Design review of the part built by this model. Coordinates are the model's own, in mm. A direction names the side the tool comes from. Coordinates: 2 decimals unless noted, no trailing zeros.
Q1. The part is to be moulded in two halves that separate along X. For faces 4 (the cylindrical face through (8.672, 11.794, 5.267)), 5 (the flat face through (-13, 0, 5)), 6 (the flat face through (-5, 0, 13)), say which applies: released by +X, released by -X, zero draft, split by the parting line, or undercut.
Q2. For faces 1 (the flat face through (-5, 15, 12)), 2 (the cylindrical face through (-5.351, -21.323, 5.429)), 3 (the flat face through (9.4, 1.4, 10)), list the 3-axis set-ups (+Z, -Z, +X, -X, +Y, -Y) from which the entire face can be reached by the end or side of a thin tool; tool diameter is ignored.
Q3. For L1, parallel to X at y = 2, z = 6.75; L2, parallel to Z at x = -10.75, y = -18.5; L3, parallel to Y at x = -5, z = 6.25, list the stretches that pass through material, from the lowest coordinate up.
Q4. For pin 1 Ø3 at (x, y) = (-5, 24) entering from +Z; pin 2 Ø1.3 at (y, z) = (4, 11.5) entering from -X; pin 3 Ø1.5 at (x, z) = (8, 6.5) entering from +Y; pin 4 Ø2 at (x, z) = (7, 6.5) entering from +Y, all flat-tipped, find the tip position at first contact; note any pin that passes through.
Q5. Take a section at A-A, the plane x = -5. State how many separate pieces and enclosed holes the cut face has, plus the area to 3 significant figures.
from build123d import *

# Parameters (mm, degrees)
SKETCH1_R           = 2.7
BOSS_EXTRUDE1_DEPTH = 11
SKETCH2_W           = 6.5
SKETCH2_H           = 30
BOSS_EXTRUDE2_DEPTH = 2
SKETCH3_W           = 7.8
SKETCH3_H           = 35.5
BOSS_EXTRUDE3_DEPTH = 1
FILLET1_R           = 5
FILLET2_R           = 0.45
FILLET3_R           = 0.8
FILLET4_R           = 0.65
FILLET5_R           = 1.85
CHAMFER1_SIZE       = 0.4


with BuildPart() as part:
    # Sketch1 → Boss-Extrude1 (new body)
    with BuildSketch(Plane.XY):
        Polygon((-13, -30), (-13, 30), (13, 28.375), (13, -28.375), align=None)
        with Locations((-5, -24)):
            Circle(SKETCH1_R, mode=Mode.SUBTRACT)
        with Locations((-5, 24)):
            Circle(SKETCH1_R, mode=Mode.SUBTRACT)
        Polygon((3.2, -17.75), (3.2, -12.35), (9.2, -12.35), (9.2, 12.35), (3.2, 12.35), (3.2, 17.75), (4.5, 17.75), (4.5, 15.547994765), (5.34, 14.15), (8.29, 14.15), (9.79, 15.65), (11, 15.65), (11, -15.65), (9.79, -15.65), (8.29, -14.15), (5.34, -14.15), (4.5, -15.547994765), (4.5, -17.75), align=None, mode=Mode.SUBTRACT)
    extrude(amount=BOSS_EXTRUDE1_DEPTH)

    # Sketch2 → Boss-Extrude2 (add)
    with BuildSketch(Plane.XY.offset(11)):
        with Locations((-5, 0)):
            Rectangle(SKETCH2_W, SKETCH2_H)
    extrude(amount=BOSS_EXTRUDE2_DEPTH)

    # Sketch3 → Boss-Extrude3 (add)
    with BuildSketch(Plane.XY.offset(11)):
        with Locations((7.1, 0)):
            Rectangle(SKETCH3_W, SKETCH3_H)
    extrude(amount=-BOSS_EXTRUDE3_DEPTH)

    # Fillet1
    fillet1_edges = [part.edges().sort_by_distance(p)[0] for p in [
        (-13, -30, 5.5),
        (-13, 30, 5.5),
        (13, 28.375, 5.5),
        (13, -28.375, 5.5),
    ]]
    fillet(fillet1_edges, radius=FILLET1_R)

    # Fillet2
    fillet2_edges = [part.edges().sort_by_distance(p)[0] for p in [
        (3.2, 17.75, 5),
        (4.5, 17.75, 5),
        (4.5, -17.75, 5),
        (3.2, -17.75, 5),
    ]]
    fillet(fillet2_edges, radius=FILLET2_R)

    # Fillet3
    fillet3_edges = [part.edges().sort_by_distance(p)[0] for p in [
        (5.34, 14.15, 5),
        (5.34, -14.15, 5),
        (-8.25, 15, 12),
        (-8.25, -15, 12),
        (-1.75, -15, 12),
        (-1.75, 15, 12),
    ]]
    fillet(fillet3_edges, radius=FILLET3_R)

    # Fillet4
    fillet4_edges = [part.edges().sort_by_distance(p)[0] for p in [
        (3.2, 12.35, 5),
        (3.2, -12.35, 5),
    ]]
    fillet(fillet4_edges, radius=FILLET4_R)

    # Fillet5
    fillet5_edges = [part.edges().sort_by_distance(p)[0] for p in [
        (9.2, -12.35, 5),
        (9.2, 12.35, 5),
    ]]
    fillet(fillet5_edges, radius=FILLET5_R)

    # Chamfer1
    chamfer1_edges = [part.edges().sort_by_distance(p)[0] for p in [
        (-7.7, -24, 0),
        (-7.7, -24, 11),
        (0.311891431, -29.168006786, 0),
        (0.311891431, -29.168006786, 11),
        (-13, 0, 0),
        (0.311891431, 29.168006786, 0),
        (13, 0, 0),
        (-11.423488195, 28.321880084, 0),
        (11.644136191, 27.101232088, 0),
        (11.644136191, -27.101232088, 0),
        (-11.423488195, -28.321880084, 0),
        (-13, 0, 11),
        (13, 0, 11),
        (0.311891431, 29.168006786, 11),
        (-11.423488195, 28.321880084, 11),
        (-7.7, 24, 0),
        (11.644136191, 27.101232088, 11),
        (11.644136191, -27.101232088, 11),
        (-11.423488195, -28.321880084, 11),
        (-7.7, 24, 11),
        (3.85, 17.75, 0),
        (3.2, 15.15, 0),
        (3.85, -17.75, 0),
        (4.5, -16.423997383, 0),
        (4.368198052, 17.618198052, 0),
        (3.331801948, 17.618198052, 0),
        (4.368198052, -17.618198052, 0),
        (3.331801948, -17.618198052, 0),
        (-5, -15, 13),
        (-8.25, 0, 13),
        (-1.75, 0, 13),
        (-5, 15, 13),
        (-1.984314575, -14.765685425, 13),
        (-8.015685425, 14.765685425, 13),
        (-1.984314575, 14.765685425, 13),
        (-8.015685425, -14.765685425, 13),
        (7.041309111, -14.15, 0),
        (4.803442191, 15.042982153, 0),
        (5.398679374, -14.253715443, 0),
        (5.398679374, 14.253715443, 0),
        (5.6, 12.35, 0),
        (3.2, -15.15, 0),
        (3.390380592, 12.540380592, 0),
        (3.390380592, -12.540380592, 0),
        (9.2, 0, 0),
        (5.6, -12.35, 0),
        (8.658147545, -11.808147545, 0),
        (8.658147545, 11.808147545, 0),
        (4.803442191, -15.042982153, 0),
        (9.04, -14.9, 0),
        (10.395, -15.65, 0),
        (11, 0, 0),
        (10.395, 15.65, 0),
        (9.04, 14.9, 0),
        (7.041309111, 14.15, 0),
        (4.5, 16.423997383, 0),
    ]]
    chamfer(chamfer1_edges, length=CHAMFER1_SIZE)


solid = part.part
Responses:
1. face 4: undercut
1. face 5: released by -X
1. face 6: zero draft
2. face 1: +Z, +X, -X, +Y
2. face 2: +Z, -Z
2. face 3: -Z
3. L1: x = -13 to 9.2, 11 to 13
3. L2: z = 0 to 11
3. L3: y = -29.5 to -26.7, -21.3 to 21.3, 26.7 to 29.5
4. pin 1: passes through
4. pin 2: stops at x = -12.75
4. pin 3: stops at y = 28.73
4. pin 4: stops at y = 28.81
5. separate pieces: 3
5. enclosed holes: 0
5. area: 589 mm2
